from build123d import *

# Parameters (mm, degrees)
F0_W      = 406.4
F0_H      = 101.6
F1_DEPTH  = 25.4
F2_W      = 50.8
F2_H      = 101.6
F3_DEPTH  = 508
F4_W      = 406.4
F4_H      = 101.6
F5_DEPTH  = 50.8
F6_W      = 406.4
F6_H      = 609.6
F7_DEPTH  = 25.4
F8_W      = 406.4
F8_H      = 50.8
F9_DEPTH  = 203.2
F10_W     = 406.4
F10_H     = 50.8
F11_DEPTH = 101.6
F12_W     = 406.4
F12_H     = 50.8
F13_DEPTH = 203.2
F14_W     = 406.4
F14_H     = 50.8
F15_DEPTH = 101.6
F17_DEPTH = 203.2
F18_W     = 812.8
F18_H     = 50.8
F19_DEPTH = 101.6
F20_W     = 1016
F20_H     = 50.8
F21_DEPTH = 203.2
F22_W     = 812.8
F22_H     = 50.8
F23_DEPTH = 101.6


with BuildPart() as f1:
    # F0 (on Front) → F1 (new body, symmetric)
    with BuildSketch(Plane.XZ):
        Rectangle(F0_W, F0_H)
    extrude(amount=F1_DEPTH, both=True)

    # F2 (on face) → F3 (join)
    with BuildSketch(Plane(origin=(0, 25.4, 0), x_dir=(-1, 0, 0), z_dir=(0, 1, 0))):
        with Locations((-177.8, 0)):
            Rectangle(F2_W, F2_H)
        with Locations((177.8, 0)):
            Rectangle(F2_W, F2_H)
    extrude(amount=F3_DEPTH)

    # F4 (on face) → F5 (join)
    with BuildSketch(Plane(origin=(0, 533.4, 0), x_dir=(-1, 0, 0), z_dir=(0, 1, 0))):
        Rectangle(F4_W, F4_H)
    extrude(amount=F5_DEPTH)

    # F6 (on face) → F7 (join)
    with BuildSketch(Plane(origin=(0, 0, -50.8), x_dir=(1, 0, 0), z_dir=(0, 0, -1))):
        with Locations((0, -279.4)):
            Rectangle(F6_W, F6_H)
    extrude(amount=F7_DEPTH)

    # F8 (on face) → F9 (join)
    with BuildSketch(Plane.XZ.offset(25.4)):
        with Locations((0, -50.8)):
            Rectangle(F8_W, F8_H)
    extrude(amount=F9_DEPTH)

    # F10 (on face) → F11 (join)
    with BuildSketch(Plane.XZ.offset(25.4)):
        Rectangle(F10_W, F10_H)
    extrude(amount=F11_DEPTH)

    # F12 (on face) → F13 (join)
    with BuildSketch(Plane(origin=(0, 584.2, 0), x_dir=(-1, 0, 0), z_dir=(0, 1, 0))):
        with Locations((0, -50.8)):
            Rectangle(F12_W, F12_H)
    extrude(amount=F13_DEPTH)

    # F14 (on face) → F15 (join)
    with BuildSketch(Plane(origin=(0, 584.2, 0), x_dir=(-1, 0, 0), z_dir=(0, 1, 0))):
        Rectangle(F14_W, F14_H)
    extrude(amount=F15_DEPTH)

    # F16 (on face) → F17 (join)
    with BuildSketch(Plane.YZ.offset(203.2)):
        Polygon((-127, -25.4), (-228.6, -25.4), (-228.6, -76.2), (787.4, -76.2), (787.4, -25.4), (685.8, -25.4), align=None)
    extrude(amount=F17_DEPTH)

    # F18 (on face) → F19 (join)
    with BuildSketch(Plane.YZ.offset(203.2)):
        with Locations((279.4, 0)):
            Rectangle(F18_W, F18_H)
    extrude(amount=F19_DEPTH)

    # F20 (on face) → F21 (join)
    with BuildSketch(Plane(origin=(-203.2, 0, 0), x_dir=(0, -1, 0), z_dir=(-1, 0, 0))):
        with Locations((-279.4, -50.8)):
            Rectangle(F20_W, F20_H)
    extrude(amount=F21_DEPTH)

    # F22 (on face) → F23 (join)
    with BuildSketch(Plane(origin=(-203.2, 0, 0), x_dir=(0, -1, 0), z_dir=(-1, 0, 0))):
        with Locations((-279.4, 0)):
            Rectangle(F22_W, F22_H)
    extrude(amount=F23_DEPTH)


solid = f1.part
The listing builds one solid part. Answer for the finished solid, in the listing's coordinates (mm). A direction names the side the tool comes from. Coordinates: 2 decimals unless noted, no trailing zeros. Order: outer loops, then holes, each group sorted by start corner. A loop starts at its lowest first (then second) coordinate and runs counter-clockwise, first axis right, second up.
Q1. A cutting plane is placed at A-A, the plane z = 6. Write down the section's boundary in (x, y).
Q2. A cutting plane is placed at B-B, the plane y = -10. Write down the section's boundary in (x, z).
Q3. Given P1, Ø10, axis at y = -125.5, z = 11.5, coming from the +X side; P2, Ø15, axis at y = 254.5, z = -4.5, coming from the -X side; P3, Ø5, axis at x = -259.5, y = 356.5, coming from the +Z side, each flat-ended and moving along its own axis, determine where each tip first touches the part or whether it passes through.
Q4. Consider line 1 (Y direction, x = -68, z = -16.5); line 2 (X direction, y = 135, z = 17.5); line 3 (X direction, y = 60.5, z = 28.5). Determine where each line is inside the solid, lowest interval first.
Q5. A cutting plane is placed at C-C, the plane x = -251. Write down the section's boundary in (y, z), and give its area (3 significant figures).
Q6. A cutting plane is placed at D-D, the plane x = 31. Write down the section's boundary in (y, z), and give its area (3 significant figures).
Q7. Which of the six approach directions +Z, -Z, +X, -X, +Y, -Y give full straight-line access (tool end or side, diameter ignored) to faces 1 (the face through (-3, -25.4, 38)), 2 (the face through (304.8, 274, 0)), 3 (the face through (4, 685.8, 0)), 4 (the face through (-2, 276, -50.8))?
Q8. For a pull along Y with two mould halves and no side action, classify faces 5 (the face through (203.2, 275, 38)), 6 (the face through (-2, 25.4, 1)), 7 (the face through (4, -127, 0)) as pulls with the +Y half, pulls with the -Y half, needs draft (parallel to the pull), parting line crosses it, or undercut.
Answers follow:
1. outline: (-304.8, -127) - (304.8, -127) - (304.8, 685.8) - (-304.8, 685.8) - close; hole (-152.4, 25.4) - (152.4, 25.4) - (152.4, 533.4) - (-152.4, 533.4) - close
2. outline: (-406.4, -76.2) - (406.4, -76.2) - (406.4, -25.4) - (304.8, -25.4) - (304.8, 25.4) - (203.2, 25.4) - (203.2, 50.8) - (-203.2, 50.8) - (-203.2, 25.4) - (-304.8, 25.4) - (-304.8, -25.4) - (-406.4, -25.4) - close
3. P1: stops at x = 304.8
3. P2: stops at x = -304.8
3. P3: stops at z = 25.4
4. line 1: y = -127 to 25.4, 533.4 to 685.8
4. line 2: x = -304.8 to -152.4, 152.4 to 304.8
4. line 3: x = -203.2 to -152.4, 152.4 to 203.2
5. outline: (-228.6, -76.2) - (787.4, -76.2) - (787.4, -25.4) - (685.8, -25.4) - (685.8, 25.4) - (-127, 25.4) - (-127, -25.4) - (-228.6, -25.4) - close
5. area: 92,900 mm2
6. outline: (-228.6, -76.2) - (787.4, -76.2) - (787.4, -25.4) - (685.8, -25.4) - (685.8, 25.4) - (584.2, 25.4) - (584.2, 50.8) - (533.4, 50.8) - (533.4, -50.8) - (25.4, -50.8) - (25.4, 50.8) - (-25.4, 50.8) - (-25.4, 25.4) - (-127, 25.4) - (-127, -25.4) - (-228.6, -25.4) - close
6. area: 56,800 mm2
7. face 1: +Z, +X, -X, -Y
7. face 2: +Z, +X, +Y, -Y
7. face 3: +Z, +X, -X, +Y
7. face 4: +Z
8. face 5: needs draft
8. face 6: undercut
8. face 7: pulls with the -Y half
